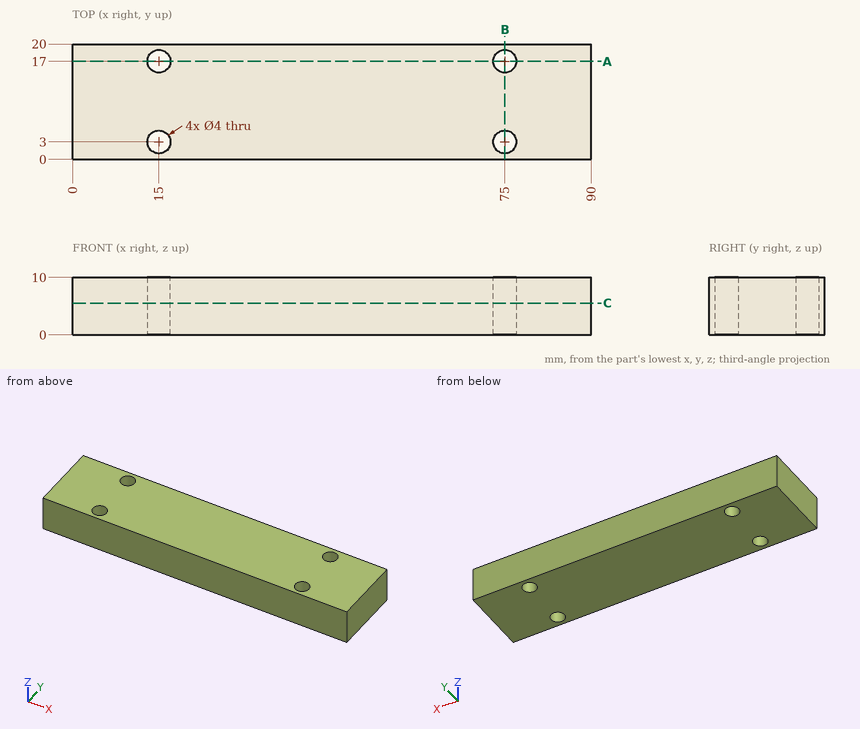
Can you work these out from the drawing? Everything is in mm from the part's minimum corner. Coordinates: 2 decimals unless noted, no trailing zeros. Loops run counter-clockwise (first coordinate to the right, second up) from the corner with the lowest first, then second, coordinate; pieces in that order, holes last.
1. Imagine slicing it at C-C, the plane z = 5.5. Please give me the cut outline in (x, y), and give its area (3 significant figures).
2. For P1, Ø4.5, axis at x = 75, y = 17, coming from the -Z side, with a flat end and sliding along its axis, tell me the tip position at first contact or that it passes through.
3. Imagine slicing it at A-A, the plane y = 17. Please give me the cut outline in (x, z), and give its area (3 significant figures).
4. Imagine slicing it at B-B, the plane x = 75. Please give me the cut outline in (y, z).
5. I need wall thicknesses on L1, parallel to Y at x = 15, z = 6.5; L2, parallel to X at y = 18.75, z = 2.5; L3, parallel to X at y = 3.5, z = 7.75. Which ranges of each line are inside material? Lowest first, please.
Taken from the geometry:
1. outline: (0, 0) - (90, 0) - (90, 20) - (0, 20) - close; hole circle Ø4 at (15, 3); hole circle Ø4 at (15, 17); hole circle Ø4 at (75, 3); hole circle Ø4 at (75, 17)
1. area: 1,750 mm2
2. P1: stops at z = 0
3. outline: (0, 0) - (13, 0) - (13, 10) - (0, 10) - close; (17, 0) - (73, 0) - (73, 10) - (17, 10) - close; (77, 0) - (90, 0) - (90, 10) - (77, 10) - close
3. area: 820 mm2
4. outline: (0, 0) - (1, 0) - (1, 10) - (0, 10) - close; (5, 0) - (15, 0) - (15, 10) - (5, 10) - close; (19, 0) - (20, 0) - (20, 10) - (19, 10) - close
5. L1: y = 0 to 1, 5 to 15, 19 to 20
5. L2: x = 0 to 14.03, 15.97 to 74.03, 75.97 to 90
5. L3: x = 0 to 13.06, 16.94 to 73.06, 76.94 to 90
